from build123d import *

# Parameters (mm, degrees)
PAD_DEPTH       = 8
FILLET_R        = 3.5
PAD001_DEPTH    = 2.5
PAD002_DEPTH    = 10
SKETCH002_R     = 1.607891
POCKET_DEPTH    = 5
POCKET001_DEPTH = 2.501
SKETCH004_W     = 33.802838
SKETCH004_H     = 3.098588
POCKET002_DEPTH = 5


with BuildPart() as obj1:
    # Sketch → Pad (new body)
    with BuildSketch(Plane.XY):
        with BuildLine():
            ThreePointArc((-29.5, 80), (-34.449747, 77.949747), (-36.5, 73))
            Line((-36.5, -73), (-36.5, 73))
            ThreePointArc((-36.5, -73), (-34.449747, -77.949747), (-29.5, -80))
            Line((29.5, -80), (-29.5, -80))
            ThreePointArc((29.5, -80), (34.449747, -77.949747), (36.5, -73))
            Line((36.5, 73), (36.5, -73))
            ThreePointArc((36.5, 73), (34.449747, 77.949747), (29.5, 80))
            Line((-29.5, 80), (29.5, 80))
        make_face()
    extrude(amount=PAD_DEPTH)

    # Fillet
    fillet_edges = [obj1.edges().sort_by_distance(p)[0] for p in [
        (-34.449747, 77.949747, 8),
        (-36.5, 0, 8),
        (-34.449747, -77.949747, 8),
        (0, -80, 8),
        (34.449747, -77.949747, 8),
        (36.5, 0, 8),
        (34.449747, 77.949747, 8),
        (0, 80, 8),
        (-34.449747, 77.949747, 0),
        (-36.5, 0, 0),
        (-34.449747, -77.949747, 0),
        (0, -80, 0),
        (34.449747, -77.949747, 0),
        (36.5, 0, 0),
        (34.449747, 77.949747, 0),
        (0, 80, 0),
    ]]
    fillet(fillet_edges, radius=FILLET_R)

    # Sketch001 (on Face11 of Fillet) → Pad001 (join, symmetric)
    with BuildSketch(Plane.XY.offset(8)):
        with BuildLine():
            ThreePointArc((-29.5, 78.25), (-33.212311, 76.712311), (-34.75, 73))
            Line((-34.75, -73), (-34.75, 73))
            ThreePointArc((-34.75, -73), (-33.212311, -76.712311), (-29.5, -78.25))
            Line((29.5, -78.25), (-29.5, -78.25))
            ThreePointArc((29.5, -78.25), (33.212311, -76.712311), (34.75, -73))
            Line((34.75, 73), (34.75, -73))
            ThreePointArc((34.75, 73), (33.212311, 76.712311), (29.5, 78.25))
            Line((-29.5, 78.25), (29.5, 78.25))
        make_face()
    extrude(amount=PAD001_DEPTH, both=True)


with BuildPart() as casebody:
    # Binder → Pad002 (new body)
    with BuildSketch(Plane(origin=(0, 0, 7.5), x_dir=(0, 1, 0), z_dir=(0, 0, 1))):
        with BuildLine():
            ThreePointArc((83.25, 29.5), (80.247845, 36.747845), (73, 39.75))
            Line((73, 39.75), (-73, 39.75))
            ThreePointArc((-73, 39.75), (-80.247845, 36.747845), (-83.25, 29.5))
            Line((-83.25, 29.5), (-83.25, -29.5))
            ThreePointArc((-83.25, -29.5), (-80.247845, -36.747845), (-73, -39.75))
            Line((-73, -39.75), (73, -39.75))
            ThreePointArc((73, -39.75), (80.247845, -36.747845), (83.25, -29.5))
            Line((83.25, -29.5), (83.25, 29.5))
        make_face()
    extrude(amount=-PAD002_DEPTH)

    # Boolean: cut obj1
    add(obj1.part, mode=Mode.SUBTRACT)

    # Sketch002 (on Face9 of Boolean) → Pocket (cut)
    with BuildSketch(Plane.XZ.offset(83.25)):
        with Locations((-24.328213, 3.143363)):
            Circle(SKETCH002_R)
        with Locations((20.529039, 3.143363)):
            Circle(SKETCH002_R)
        with BuildLine():
            ThreePointArc((-6.939364, 5.148021), (-8.944022, 3.143363), (-6.939364, 1.138705))
            Line((-6.939364, 1.138705), (6.939364, 1.138705))
            ThreePointArc((6.939364, 1.138705), (8.944022, 3.143363), (6.939364, 5.148021))
            Line((6.939364, 5.148021), (-6.939364, 5.148021))
        make_face()
    extrude(amount=-POCKET_DEPTH, mode=Mode.SUBTRACT)

    # Sketch003 (on Face44 of Pocket) → Pocket001 (cut, through all)
    with BuildSketch(Plane.XY):
        with BuildLine():
            ThreePointArc((-22.971405, 66.593148), (-26.905647, 64.963532), (-28.535263, 61.02929))
            Line((-28.535263, 48.647752), (-28.535263, 61.02929))
            ThreePointArc((-28.535263, 48.647752), (-26.905647, 44.71351), (-22.971405, 43.083894))
            Line((-11.843698, 43.083894), (-22.971405, 43.083894))
            ThreePointArc((-11.843698, 43.083894), (-7.909456, 44.71351), (-6.27984, 48.647752))
            Line((-6.27984, 61.02929), (-6.27984, 48.647752))
            ThreePointArc((-6.27984, 61.02929), (-7.909456, 64.963532), (-11.843698, 66.593148))
            Line((-22.971405, 66.593148), (-11.843698, 66.593148))
        make_face()
    extrude(amount=-POCKET001_DEPTH, mode=Mode.SUBTRACT)

    # Sketch004 (on Face8 of Pocket001) → Pocket002 (cut)
    with BuildSketch(Plane.YZ.offset(39.75)):
        with Locations((48.748877, 1.369124)):
            Rectangle(SKETCH004_W, SKETCH004_H)
    extrude(amount=-POCKET002_DEPTH, mode=Mode.SUBTRACT)


solid = casebody.part
Design review of the part built by this model. Coordinates are the model's own, in mm. A direction names the side the tool comes from. Give positions to 0.01 mm unless a question says otherwise; leave off trailing zeros. Loops run counter-clockwise (first coordinate to the right, second up) from the corner with the lowest first, then second, coordinate; pieces in that order, holes last. Notation, with made-up numbers: (34.25, 12) -> (69.25, 12) arc R29 cw to (69.25, 40) -> close; hole circle Ø9 at (88, -20). An arc over 180 degrees is marked (long way). One line per question, with ' | ' between items. Start each with the question number.
(1) For faces 4 (the face through (-7.953, 44.67, -1.232)), 5 (the face through (0, 1, 0)), 6 (the face through (38, 31.847, 1)), 7 (the face through (-34.5, -77.9, 4)), list the 3-axis set-ups (+Z, -Z, +X, -X, +Y, -Y) from which the entire face can be reached by the end or side of a thin tool; tool diameter is ignored.
(2) We need section B-B (y = -14.5). State the section outline as (x, z) points.
(3) Draft analysis for pull direction Y (two halves, no side actions). For faces 1 (the face through (36.668, -80.327, 2.57)), 2 (the face through (-1, -1, -2.5)), 3 (the face through (38, 65.65, 1)), state which applies: +Y half, -Y half, draft (parallel to the pull), parting line (faces both ways), or undercut.
(4) We need section D-D (x = 13). State the section outline as (y, z) points.
(5) For line 1 (X direction, y = 58, z = -0.25); line 2 (X direction, y = -65.5, z = 3.5); line 3 (Y direction, x = -29, z = 5), list the stretches that pass through material, from the lowest coordinate up.
(6) Insertion check: P1, Ø2.5, axis at x = 37.5, z = 1.5, coming from the -Y side; P2, Ø1, axis at x = -31, z = 1.5, coming from the +Y side; P3, Ø1.5, axis at x = 23, y = 7, coming from the +Z side. Each pin has a flat end and moves straight along its axis. Give the tip position at first contact, or say it passes through.
(7) We need section C-C (y = 59.5). State the section outline as (x, z) points, and give its area (3 significant figures).
(8) We need section A-A (x = -17). State the section outline as (y, z) points, and give its area (3 significant figures).
The answers:
1) face 4: +Z, -Z | face 5: +Z | face 6: +X | face 7: none
2) outline: (-39.75, -2.5) -> (39.75, -2.5) -> (39.75, 7.5) -> (34.8, 7.5) arc R3.5 cw to (36.5, 4.5) -> (36.5, 3.5) arc R3.5 cw to (33, 0) -> (-33, 0) arc R3.5 cw to (-36.5, 3.5) -> (-36.5, 4.5) arc R3.5 cw to (-34.8, 7.5) -> (-39.75, 7.5) -> close
3) face 1: -Y half | face 2: draft | face 3: undercut
4) outline: (-83.25, -2.5) -> (83.25, -2.5) -> (83.25, 7.5) -> (78.3, 7.5) arc R3.5 cw to (80, 4.5) -> (80, 3.5) arc R3.5 cw to (76.5, 0) -> (-76.5, 0) arc R3.5 cw to (-80, 3.5) -> (-80, 4.5) arc R3.5 cw to (-78.3, 7.5) -> (-83.25, 7.5) -> close
5) line 1: x = -39.75 to -28.54, -6.28 to 39.75 | line 2: x = -39.75 to -36.5, 36.5 to 39.75 | line 3: y = -83.25 to -79.96, 79.96 to 83.25
6) P1: stops at y = -80.71 | P2: stops at y = 83.2 | P3: stops at z = 0
7) outline: (-39.75, -2.5) -> (-28.54, -2.5) -> (-28.54, 0) -> (-33, 0) arc R3.5 cw to (-36.5, 3.5) -> (-36.5, 4.5) arc R3.5 cw to (-34.8, 7.5) -> (-39.75, 7.5) -> close; (-6.28, -2.5) -> (39.75, -2.5) -> (39.75, -0.18) -> (34.75, -0.18) -> (34.75, 0.47) arc R3.5 cw to (33, 0) -> (-6.28, 0) -> close; (34.8, 7.5) arc R3.5 cw to (36.5, 4.5) -> (36.5, 3.5) arc R3.5 cw to (36.45, 2.92) -> (39.75, 2.92) -> (39.75, 7.5) -> close | area: 187 mm^2
8) outline: (-83.25, -2.5) -> (43.08, -2.5) -> (43.08, 0) -> (-76.5, 0) arc R3.5 cw to (-80, 3.5) -> (-80, 4.5) arc R3.5 cw to (-78.3, 7.5) -> (-83.25, 7.5) -> close; (66.59, -2.5) -> (83.25, -2.5) -> (83.25, 7.5) -> (78.3, 7.5) arc R3.5 cw to (80, 4.5) -> (80, 3.5) arc R3.5 cw to (76.5, 0) -> (66.59, 0) -> close | area: 414 mm^2
